```python
from build123d import *

# Parameters (mm, degrees)
SKETCH1_W           = 100
SKETCH1_H           = 120
BOSS_EXTRUDE1_DEPTH = 5
SKETCH2_R           = 5
SKETCH2_R_2         = 2.5
BOSS_EXTRUDE2_DEPTH = 50


with BuildPart() as part:
    # Sketch1 → Boss-Extrude1 (new, symmetric)
    with BuildSketch(Plane(origin=(0, 0, 0), x_dir=(1, 0, 0), z_dir=(0, 1, 0))):
        Rectangle(SKETCH1_W, SKETCH1_H)
    extrude(amount=BOSS_EXTRUDE1_DEPTH, both=True)

    # Sketch2 → Boss-Extrude2 (add)
    with BuildSketch(Plane(origin=(0, 5, 0), x_dir=(1, 0, 0), z_dir=(0, 1, 0))):
        with Locations(Location((-17.75, 30, 0), (0, 0, 270))):
            Circle(SKETCH2_R)
        with Locations(Location((17.75, 30, 0), (0, 0, 90))):
            Circle(SKETCH2_R)
        with Locations(Location((-12.5, -30, 0), (0, 0, 270))):
            Circle(SKETCH2_R_2)
        with Locations(Location((12.5, -30, 0), (0, 0, 270))):
            Circle(SKETCH2_R_2)
    extrude(amount=BOSS_EXTRUDE2_DEPTH)


solid = part.part
```
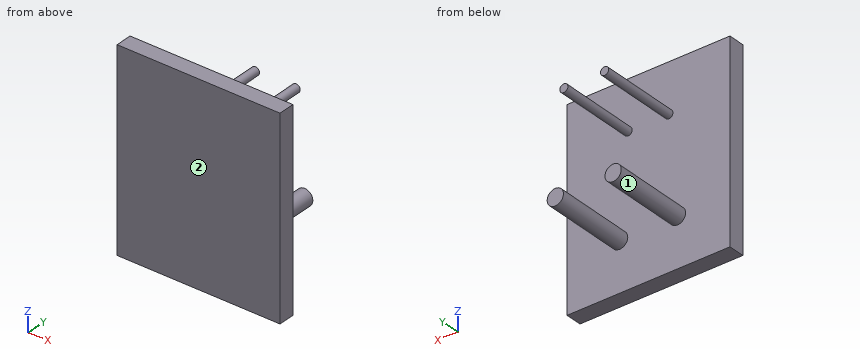
Geometry: final body of the model. Coordinates: model frame, mm. Face numbers are marked on the shaded views. Give positions to 0.01 mm unless a question says otherwise; leave off trailing zeros. Loops run counter-clockwise (first coordinate to the right, second up) from the corner with the lowest first, then second, coordinate; pieces in that order, holes last. Notation, with made-up numbers: (89, 40) -> (95, 40) arc R26 ccw to (95, 73) -> close; hole circle Ø8 at (-15, 0.25). An arc over 180 degrees is marked (long way). Use CSV: the item, a comma, the result in double quotes.
(1) Cut plane C-C (z = -30). Output: boundary loops of the cut face in (x, y).
From the geometry:
outline,"(-50, -5) -> (50, -5) -> (50, 5) -> (22.75, 5) -> (22.75, 55) -> (12.75, 55) -> (12.75, 5) -> (-12.75, 5) -> (-12.75, 55) -> (-22.75, 55) -> (-22.75, 5) -> (-50, 5) -> close"
(2) Cut plane B-B (y = 50.5). Output: boundary loops of the cut face in (x, z).
From the geometry:
outline,"circle Ø10 at (-17.75, -30); circle Ø5 at (-12.5, 30); circle Ø5 at (12.5, 30); circle Ø10 at (17.75, -30)"
(3) Ray query, line 1 along Y through (x, z) = (-2.5, -24); line 2 along X through (y, z) = (5.5, 28); line 3 along Z through (x, y) = (-17, 13). Return the intervals inside material, ascending. Write a range as [from, to].
From the geometry:
line 1,"[-5, 5]"
line 2,"[-14, -11], [11, 14]"
line 3,"[-34.94, -25.06]"
(4) Pull-direction query (X, two-part tool) for the marked faces 1 and 2; classes: released by +X, released by -X, zero draft, split by the parting line, or undercut.
From the geometry:
face 1,"undercut"
face 2,"zero draft"
(5) Cut plane A-A (x = -17.75). Output: boundary loops of the cut face in (y, z).
From the geometry:
outline,"(-5, -60) -> (5, -60) -> (5, -35) -> (55, -35) -> (55, -25) -> (5, -25) -> (5, 60) -> (-5, 60) -> close"
(6) First-contact query: P1, Ø6, axis at x = -11.5, y = 42.5, coming from the +Z side; P2, Ø12, axis at x = 7.5, y = 42, coming from the -Z side; P3, Ø2, axis at x = -4.5, z = 16, coming from the +Y side. Flat tips, straight axial feed; report the tip coordinate or a pass-through.
From the geometry:
P1,"z = 32.5"
P2,"z = -32.63"
P3,"y = 5"
(7) Cut plane D-D (z = 30). Output: boundary loops of the cut face in (x, y), plus the area to 3 significant figures.
From the geometry:
outline,"(-50, -5) -> (50, -5) -> (50, 5) -> (15, 5) -> (15, 55) -> (10, 55) -> (10, 5) -> (-10, 5) -> (-10, 55) -> (-15, 55) -> (-15, 5) -> (-50, 5) -> close"
area,"1,500 mm^2"
